Work out the finished part from the listing and answer in its coordinate system (mm). A direction names the side the tool comes from. Give positions to 0.01 mm unless a question says otherwise; leave off trailing zeros. Write each loop counter-clockwise with the first axis right and the second up, starting at its lowest first coordinate (ties: lowest second). Pieces come first, ordered by that corner, then holes. Notation, with made-up numbers: (88, 82.5) - (115, 82.5) arc R14 cw to (115, 93.5) - close; hole circle Ø8 at (42.5, -8.5). An arc over 180 degrees is marked (long way). Write item = value, one per line.
from build123d import *

# Parameters (mm, degrees)
F0_R     = 9.5463982086
F0_R_2   = 10.1052061562
F1_DEPTH = 25
F2_T     = -2.5


with BuildPart() as f1:
    # F0 (on Front) → F1 (new body)
    with BuildSketch(Plane.XZ):
        with BuildLine():
            ThreePointArc((-63.3736327291, -19.9749078602), (-2.6254435723, -20.5386626808), (58.1239726957, -20.1278970252))
            ThreePointArc((58.1239726957, -20.1278970252), (59.2157785581, 17.7962266983), (43.5713953632, 52.3604346985))
            ThreePointArc((43.5713953632, 52.3604346985), (-3.7218306533, 52.7863086545), (-51.0150566697, 52.3604346985))
            ThreePointArc((-51.0150566697, 52.3604346985), (-69.4086528725, 31.8843311692), (-63.3736327291, 5.029653199))
            ThreePointArc((-63.3736327291, 5.029653199), (-63.743030193, -7.4726273306), (-63.3736327291, -19.9749078602))
        make_face()
        with Locations((-45.056629926, 13.0809573457)):
            Circle(F0_R, mode=Mode.SUBTRACT)
        with Locations((0, 10.1740779355)):
            Circle(F0_R_2, mode=Mode.SUBTRACT)
    extrude(amount=F1_DEPTH)

    # F2
    f2_openings = [f1.faces().sort_by_distance(p)[0] for p in [
        (-2.62355, -25, -19.035238),
    ]]
    offset(amount=F2_T, openings=f2_openings, kind=Kind.INTERSECTION)


solid = f1.part
1. Find section B-B, the plane x = -49. Give the vertices of the cut face in (y, z), then the cut area to 3 significant figures.
Solution:
outline = (-25, -20.2) - (0, -20.2) - (0, 4.39) - (-25, 4.39) - (-25, 1.7) - (-2.5, 1.7) - (-2.5, -17.7) - (-25, -17.7) - close; (-25, 21.77) - (0, 21.77) - (0, 52.4) - (-25, 52.4) - (-25, 49.9) - (-2.5, 49.9) - (-2.5, 24.46) - (-25, 24.46) - close
area = 372 mm^2
2. Given pin 1 (1.5 mm diameter, centred on x = 38.5, z = 1.5, fed in from -Y); pin 2 (1 mm diameter, centred on x = -39.5, y = -15.5, fed in from +Z); pin 3 (6 mm diameter, centred on y = -4.5, z = 9.5, fed in from +X), each flat-ended and moving along its own axis, determine where each tip first touches the part or whether it passes through.
Solution:
pin_1 = -2.5
pin_2 = 52.55
pin_3 = 60.7
3. Find section D-D, the plane z = 46.5. Give the vertices of the cut face in (x, y), then the cut area to 3 significant figures.
Solution:
outline = (-60.57, -25) - (-56.62, -25) - (-56.62, -2.5) - (44.68, -2.5) - (44.68, -25) - (47.66, -25) - (47.66, 0) - (-60.57, 0) - close
area = 426 mm^2
4. A tool of negligible diameter and unlimited length cuts with its end or side. For faces 5 (the cylindrical face through (-61.235, -13.592, -5.643)), 6 (the cylindrical face through (-3.476, -12.325, -20.537)), 7 (the cylindrical face through (-3.06, -12.325, 52.786)), from which of +Z, -Z, +X, -X, +Y, -Y can it reach the whole face along a straight path? Write none if from no direction.
Solution:
face_5 = -Y
face_6 = -Z, +Y, -Y
face_7 = +Z, +Y, -Y
5. Find section A-A, the plane y = -11.75. Give the vertices of the cut face in (x, z).
Solution:
outline = (-63.37, -19.97) arc R3787.15 ccw to (58.12, -20.13) arc R84.32 ccw to (43.57, 52.36) arc R2626.17 ccw to (-51.02, 52.36) arc R30.01 ccw to (-63.37, 5.03) arc R211.75 ccw to start; circle Ø24.09 at (-45.06, 13.08); circle Ø25.21 at (0, 10.17); hole (-61, -17.51) arc R3784.65 ccw to (56.16, -17.66) arc R81.82 ccw to (42.31, 49.88) arc R2623.67 ccw to (-50.53, 49.87) arc R27.51 ccw to (-60.82, 5.9) arc R209.25 ccw to start; hole circle Ø19.09 at (-45.06, 13.08); hole circle Ø20.21 at (0, 10.17)
6. Straight lines are drawn through the part: line 1 (Z direction, x = 0, y = -7.75); line 2 (X direction, y = -11, z = 20.5); line 3 (Z direction, x = -1, y = -16.75). For each, find the intervals that lie inside material, in ascending order.
Solution:
line_1 = -20.54 to -18.04, -2.43 to 0.07, 20.28 to 22.78, 50.28 to 52.78
line_2 = -70.14 to -67.62, -54.55 to -51.06, -39.05 to -35.57, -7.23 to 7.23, 56.06 to 58.63
line_3 = -20.54 to -18.04, -2.39 to 0.12, 20.23 to 22.74, 50.28 to 52.78
7. Find section C-C, the plane z = 7.5. Give the vertices of the cut face in (x, y), then the cut area to 3 significant figures.
Solution:
outline = (-65.24, -25) - (-62.15, -25) - (-62.15, -2.5) - (-55.73, -2.5) - (-55.73, -25) - (-52.8, -25) - (-52.8, 0) - (-65.24, 0) - close; (-37.31, -25) - (-34.38, -25) - (-34.38, -2.5) - (-12.32, -2.5) - (-12.32, -25) - (-9.74, -25) - (-9.74, 0) - (-37.31, 0) - close; (9.74, -25) - (12.32, -25) - (12.32, -2.5) - (58.12, -2.5) - (58.12, -25) - (60.63, -25) - (60.63, 0) - (9.74, 0) - close
area = 601 mm^2
8. For a pull along X with two mould halves and no side action, classify faces 1 (the cylindrical face through (-8, -12, 4)), 2 (the flat face through (0, -25, 21)), 3 (the cylindrical face through (56.794, -13.592, 17.156)), 4 (the cylindrical face through (-69.305, -12.325, 32.271)) as pulls with the +X half, pulls with the -X half, needs draft (parallel to the pull), parting line crosses it, or undercut.
Solution:
face_1 = undercut
face_2 = needs draft
face_3 = undercut
face_4 = pulls with the -X half
